Build history of the part. All positions in model axes, mm. Round coordinates to 2 decimals unless told otherwise and drop trailing zeros. Write each loop counter-clockwise with the first axis right and the second up, starting at its lowest first coordinate (ties: lowest second). Pieces come first, ordered by that corner, then holes.
Autodesk Inventor part; units mm, degrees
ref_plane "YZ Plane" through (0, 0, 0) normal (1, 0, 0) x (0, 1, 0)
ref_plane "XZ Plane" through (0, 0, 0) normal (0, 1, 0) x (-1, 0, 0)
ref_plane "XY Plane" through (0, 0, 0) normal (0, 0, 1) x (1, 0, 0)
sketch "Эскиз1" plane through (0, 0, 0) normal (0, 1, 0) x (-1, 0, 0)
  line L0 (-200, 0) -> (-600, 0)
  line L1 (-600, 0) -> (-600, -600)
  line L2 (-600, -600) -> (-200, -600)
  line L3 (-200, 0) -> (-250, 0)
  line L4 (-250, 0) -> (-200, 0)
  line L5 (-258, -230) -> (-258, -370)
  line L6 (-300, -230) -> (-258, -230)
  line L7 (-300, -370) -> (-258, -370)
  line L8 (-258, -335) -> (-258, -265)
  line L9 (-300, 0) -> (-200, 0)
  line L10 (-258, -300) -> (-258, -247.9631)
  line L11 (-258, -300) -> (-250, -300)
  line L12 (-250, -300) -> (-250, -280)
  line L13 (-250, -280) -> (-250, -300)
  line L14 (-250, -300) -> (-250, -320)
  circle A0 centre (-250, -320) radius 3.5
  circle A1 centre (-250, -300) radius 3.5
  circle A2 centre (-250, -280) radius 3.5
  line L15 (-300, -300) -> (-300, -230)
  line L16 (-600, 0) -> (-250, 0)
  line L17 (-600, 0) -> (-200, 0)
  line L18 (-200, 0) -> (-200, -600)
  line L19 (-300, -370) -> (-300, -300)
  point P0 (0, 0)
  point P1 (-200, -600)
  point P2 (-200, 0)
  dimension "d1" = 600
  dimension "d16" = 140
  dimension "d17" = 42
  dimension "d23" = 8
  dimension "d24" = 20
  dimension "d26" = 20
  dimension "d27" = 7
  dimension "d28" = 7
  dimension "d29" = 7
  dimension "d30" = 70
  dimension "d31" = 300
  dimension "d33" = 400
extrude "Выдавливание2" add sketch "Эскиз1" along normal blind 8
properties part number "Нижняя полка"
1) Slice it at A-A (y = 5.75). Write the cut outline in (x, z).
Results:
outline: (200, -600) - (600, -600) - (600, 0) - (200, 0) - close; hole circle Ø7 at (250, -320); hole circle Ø7 at (250, -300); hole circle Ø7 at (250, -280); hole (258, -370) - (300, -370) - (300, -230) - (258, -230) - close
2) Wall check: L1, parallel to Z at x = 250, y = 6.25; L2, parallel to X at y = 2.25, z = -320; L3, parallel to X at y = 3, z = -329. Give the ranges that are in metal, low to high.
Results:
L1: z = -600 to -323.5, -316.5 to -303.5, -296.5 to -283.5, -276.5 to 0
L2: x = 200 to 246.5, 253.5 to 258, 300 to 600
L3: x = 200 to 258, 300 to 600
3) Pin check, flat tips, straight feed: pin 1 Ø2 at (x, z) = (416.5, -81.5) entering from -Y; pin 2 Ø4 at (x, z) = (250, -280) entering from -Y. Stop position of each tip, or through.
Results:
pin 1: stops at y = 0
pin 2: passes through
